Here's how the part is built. I have some questions about the finished solid (model axes, mm). Face numbers are marked on the shaded views. A direction names the side the tool comes from. Round coordinates to 2 decimals unless told otherwise and drop trailing zeros. Loops run counter-clockwise (first coordinate to the right, second up) from the corner with the lowest first, then second, coordinate; pieces in that order, holes last. Notation, with made-up numbers: (81, 50) -> (119, 50) arc R22 ccw to (119, 84) -> close; hole circle Ø5 at (83, -30). An arc over 180 degrees is marked (long way). Use CSV: the item, a comma, the result in double quotes. Start each with the question number.
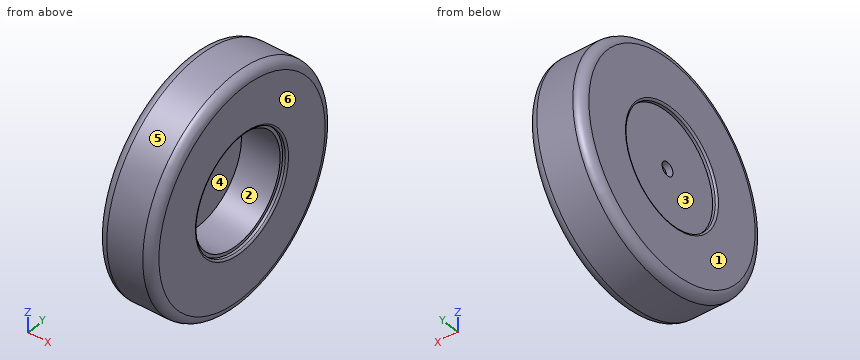
from build123d import *

# Parameters (mm, degrees)
HUB_START      = 5
SKETCH1_R      = 63.5
SKETCH1_R_2    = 7.625
HUB_FACE_DEPTH = 7
SKETCH2_R      = 63.5
SKETCH2_R_2    = 60
HUB_DEPTH      = 50
SKETCH3_R      = 127
SKETCH3_R_2    = 63.5
RUBBER_DEPTH   = 60
FILLET1_R      = 10
FILLET2_R      = 2


with BuildPart() as part:
    # Sketch1 → Hub Face (new body)
    with BuildSketch(Plane(origin=(0, 0, 0), x_dir=(0, 0, -1), z_dir=(1, 0, 0)).offset(HUB_START)):
        Circle(SKETCH1_R)
        Circle(SKETCH1_R_2, mode=Mode.SUBTRACT)
    extrude(amount=HUB_FACE_DEPTH)

    # Sketch2 → Hub (add)
    with BuildSketch(Plane(origin=(0, 0, 0), x_dir=(0, 0, -1), z_dir=(1, 0, 0)).offset(HUB_START)):
        Circle(SKETCH2_R)
        Circle(SKETCH2_R_2, mode=Mode.SUBTRACT)
    extrude(amount=HUB_DEPTH)

    # Sketch3 → Rubber (add)
    with BuildSketch(Plane(origin=(0, 0, 0), x_dir=(0, 0, -1), z_dir=(1, 0, 0))):
        Circle(SKETCH3_R)
        Circle(SKETCH3_R_2, mode=Mode.SUBTRACT)
    extrude(amount=RUBBER_DEPTH)

    # Fillet1
    fillet1_edges = [part.edges().sort_by_distance(p)[0] for p in [
        (60, 0, 127),
        (0, 0, 127),
    ]]
    fillet(fillet1_edges, radius=FILLET1_R)

    # Fillet2
    fillet2_edges = [part.edges().sort_by_distance(p)[0] for p in [
        (0, 0, 63.5),
        (60, 0, 63.5),
    ]]
    fillet(fillet2_edges, radius=FILLET2_R)


solid = part.part
Q1. I want a section at C-C, the plane x = 45. List the corners of the cut face in (y, z) for me.
Q2. If we mould it in two halves opening along Y, with no side actions, what happens to the marked faces 4, 5 and 6? For each: pulls with the +Y half, pulls with the -Y half, needs draft (parallel to the pull), parting line crosses it, or undercut.
Q3. I want a section at A-A, the plane y = 0. List the corners of the cut face in (x, z) for me (3 decimals).
Q4. For the marked faces 1, 2 and 3, which set-ups out of +Z, -Z, +X, -X, +Y, -Y let a thin tool reach every point of the face, with its end or its side?
Q5. I need wall thicknesses on line 1 along Y through (x, z) = (19, 2); line 2 along X through (y, z) = (44, 14); line 3 along Z through (x, y) = (25.5, 49). Which ranges of each line are inside material? Lowest first, please.
Q6. Will these pins go through, and if not, where does the flat tip stop? pin 1 Ø1 at (x, y) = (47.5, 50) entering from +Z; pin 2 Ø8 at (x, z) = (31, 61.5) entering from +Y; pin 3 Ø2 at (x, z) = (8, 73) entering from +Y; pin 4 Ø9 at (y, z) = (0, 0) entering from -X.
Values found:
1,outline,"circle Ø254 at (0, 0); hole circle Ø120 at (0, 0)"
2,face 4,"undercut"
2,face 5,"parting line crosses it"
2,face 6,"needs draft"
3,outline,"(0, -117) arc R10 ccw to (10, -127) -> (50, -127) arc R10 ccw to (60, -117) -> (60, -65.5) arc R2 ccw to (58, -63.5) -> (55, -63.5) -> (55, -60) -> (12, -60) -> (12, -7.625) -> (5, -7.625) -> (5, -63.5) -> (2, -63.5) arc R2 ccw to (0, -65.5) -> close; (0, 65.5) arc R2 ccw to (2, 63.5) -> (5, 63.5) -> (5, 7.625) -> (12, 7.625) -> (12, 60) -> (55, 60) -> (55, 63.5) -> (58, 63.5) arc R2 ccw to (60, 65.5) -> (60, 117) arc R10 ccw to (50, 127) -> (10, 127) arc R10 ccw to (0, 117) -> close"
4,face 1,"+Z, -Z, -X, +Y, -Y"
4,face 2,"+X"
4,face 3,"-X"
5,line 1,"-126.98 to -59.97, 59.97 to 126.98"
5,line 2,"5 to 12"
5,line 3,"-117.17 to -34.63, 34.63 to 117.17"
6,pin 1,"z = 116.96"
6,pin 2,"y = 113.24"
6,pin 3,"y = 104.41"
6,pin 4,"through"
